Geometry: final body of the model. Coordinates: model frame, mm. A direction names the side the tool comes from. Coordinates: 2 decimals unless noted, no trailing zeros. Loops run counter-clockwise (first coordinate to the right, second up) from the corner with the lowest first, then second, coordinate; pieces in that order, holes last. Notation, with made-up numbers: (-28.5, 81.5) - (17.5, 81.5) arc R27 cw to (17.5, 110.5) - close; hole circle Ø7 at (-34.75, 46.25). An arc over 180 degrees is marked (long way). Return JSON: item names as keys, results as strings.
from build123d import *

# Parameters (mm, degrees)
EXTRUDE_THIN1_DEPTH    = 16.002
CUT_EXTRUDE1_START     = -15.748
CUT_EXTRUDE1_OUTLINE_R = 1.3
CUT_EXTRUDE1_DEPTH     = 15.748
BOSS_EXTRUDE2_DEPTH    = 1.68
BOSS_EXTRUDE3_START    = 1.68
BOSS_EXTRUDE3_DEPTH    = 1.68
CUT_EXTRUDE2_START     = -2.384
CUT_EXTRUDE2_DEPTH     = 2.384
CUT_EXTRUDE3_DEPTH     = 2.384
CHAMFER1_SIZE          = 1.7
CHAMFER2_SIZE          = 2.38


# Read off the part's stored shape, not the designer's step: Cut-Extrude1
with BuildPart() as part:
    # Sketch1 → Extrude-Thin1 (new body)
    with BuildSketch(Plane.XY):
        with BuildLine():
            Line((-42.06875, -12.7), (-35.433, -12.7))
            ThreePointArc((-35.433, -12.7), (-33.636948776, -11.956051224), (-32.893, -10.16))
            Line((-32.893, -10.16), (-32.893, -2.54))
            ThreePointArc((-32.893, -2.54), (-32.149051224, -0.743948776), (-30.353, 0))
            Line((-30.353, 0), (30.353, 0))
            ThreePointArc((30.353, 0), (32.149051224, -0.743948776), (32.893, -2.54))
            Line((32.893, -2.54), (32.893, -10.16))
            ThreePointArc((32.893, -10.16), (33.636948776, -11.956051224), (35.433, -12.7))
            Line((35.433, -12.7), (42.06875, -12.7))
            Line((42.06875, -12.7), (42.06875, -15.748))
            Line((42.06875, -15.748), (35.433, -15.748))
            ThreePointArc((35.433, -15.748), (31.481687307, -14.111312693), (29.845, -10.16))
            Line((29.845, -10.16), (29.845, -3.048))
            Line((29.845, -3.048), (-29.845, -3.048))
            Line((-29.845, -3.048), (-29.845, -10.16))
            ThreePointArc((-29.845, -10.16), (-31.481687307, -14.111312693), (-35.433, -15.748))
            Line((-35.433, -15.748), (-42.06875, -15.748))
            Line((-42.06875, -15.748), (-42.06875, -12.7))
        make_face()
    extrude(amount=-EXTRUDE_THIN1_DEPTH)

    # Cut-Extrude1 outline → Cut-Extrude1 (cut)
    with BuildSketch(Plane(origin=(0, 0, 0), x_dir=(1, 0, 0), z_dir=(0, 1, 0)).offset(CUT_EXTRUDE1_START)):
        with BuildLine():
            Line((35.433, 13.462), (-35.433, 13.462))
            ThreePointArc((-35.433, 13.462), (-37.133, 11.762), (-35.433, 10.062))
            Line((-35.433, 10.062), (-32.893, 10.062))
            Line((-32.893, 10.062), (-32.893, 8.382))
            Line((-32.893, 8.382), (-1.27, 8.382))
            Line((-1.27, 8.382), (-1.27, 12.446))
            Line((-1.27, 12.446), (32.893, 12.446))
            Line((32.893, 12.446), (32.893, 10.062))
            Line((32.893, 10.062), (35.433, 10.062))
            ThreePointArc((35.433, 10.062), (37.133, 11.762), (35.433, 13.462))
        make_face()
        with BuildLine():
            Line((32.893, 5.94), (32.893, 7.62))
            Line((32.893, 7.62), (1.27, 7.62))
            Line((1.27, 7.62), (1.27, 3.556))
            Line((1.27, 3.556), (-32.893, 3.556))
            Line((-32.893, 3.556), (-32.893, 5.94))
            Line((-32.893, 5.94), (-35.433, 5.94))
            ThreePointArc((-35.433, 5.94), (-37.133, 4.24), (-35.433, 2.54))
            Line((-35.433, 2.54), (35.433, 2.54))
            ThreePointArc((35.433, 2.54), (37.133, 4.24), (35.433, 5.94))
            Line((35.433, 5.94), (32.893, 5.94))
        make_face()
        with BuildLine():
            Line((42.06875, 16.002), (35.433, 16.002))
            ThreePointArc((35.433, 16.002), (40.193949205, 13.198335352), (42.06875, 8.001))
            Line((42.06875, 8.001), (42.06875, 16.002))
        make_face()
        with BuildLine():
            Line((42.06875, 0), (42.06875, 8.001))
            ThreePointArc((42.06875, 8.001), (40.193949205, 2.803664648), (35.433, 0))
            Line((35.433, 0), (42.06875, 0))
        make_face()
        with BuildLine():
            ThreePointArc((-42.06875, 8.001), (-40.193949205, 13.198335352), (-35.433, 16.002))
            Line((-35.433, 16.002), (-42.06875, 16.002))
            Line((-42.06875, 16.002), (-42.06875, 8.001))
        make_face()
        with BuildLine():
            ThreePointArc((-35.433, 0), (-40.193949205, 2.803664648), (-42.06875, 8.001))
            Line((-42.06875, 8.001), (-42.06875, 0))
            Line((-42.06875, 0), (-35.433, 0))
        make_face()
        with Locations((38.750875, 8.001)):
            Circle(CUT_EXTRUDE1_OUTLINE_R)
        with Locations((-38.750875, 8.001)):
            Circle(CUT_EXTRUDE1_OUTLINE_R)
    extrude(amount=CUT_EXTRUDE1_DEPTH, mode=Mode.SUBTRACT)

    # Sketch6 → Boss-Extrude2 (add)
    with BuildSketch(Plane(origin=(0, 0, -8.382), x_dir=(-1, 0, 0), z_dir=(0, 0, -1))):
        with BuildLine():
            Line((32.893, -10.16), (32.893, -6.604))
            Line((32.893, -6.604), (29.845, -6.604))
            Line((29.845, -6.604), (29.845, -10.16))
            ThreePointArc((29.845, -10.16), (30.667537588, -13.078237824), (32.893, -15.137363157))
            Line((32.893, -15.137363157), (32.893, -10.16))
        make_face()
    extrude(amount=BOSS_EXTRUDE2_DEPTH)

    # Sketch7 → Boss-Extrude3 (add)
    with BuildSketch(Plane.XY.offset(-7.62).offset(BOSS_EXTRUDE3_START)):
        with BuildLine():
            Line((32.893, -10.16), (32.893, -6.6))
            Line((32.893, -6.6), (29.845, -6.604))
            Line((29.845, -6.604), (29.845, -10.16))
            ThreePointArc((29.845, -10.16), (30.667537588, -13.078237824), (32.893, -15.137363157))
            Line((32.893, -15.137363157), (32.893, -10.16))
        make_face()
    extrude(amount=-BOSS_EXTRUDE3_DEPTH)

    # Sketch8 → Cut-Extrude2 (cut)
    with BuildSketch(Plane(origin=(0, 0, -12.446), x_dir=(-1, 0, 0), z_dir=(0, 0, -1)).offset(CUT_EXTRUDE2_START)):
        with BuildLine():
            Line((-32.893, -15.137363157), (-32.893, -6.6))
            Line((-32.893, -6.6), (-29.845, -6.604))
            Line((-29.845, -6.604), (-29.845, -10.16))
            ThreePointArc((-29.845, -10.16), (-30.667537588, -13.078237824), (-32.893, -15.137363157))
        make_face()
    extrude(amount=CUT_EXTRUDE2_DEPTH, mode=Mode.SUBTRACT)

    # Sketch9 → Cut-Extrude3 (cut)
    with BuildSketch(Plane.XY.offset(-3.556)):
        with BuildLine():
            Line((-32.893, -15.137363157), (-32.893, -6.604))
            Line((-32.893, -6.604), (-29.845, -6.604))
            Line((-29.845, -6.604), (-29.845, -10.16))
            ThreePointArc((-29.845, -10.16), (-30.667537588, -13.078237824), (-32.893, -15.137363157))
        make_face()
    extrude(amount=-CUT_EXTRUDE3_DEPTH, mode=Mode.SUBTRACT)

    # Chamfer1
    # the kernel refuses this chamfer: 1.7 mm, written as the material it adds along each edge
    # the kernel refuses this chamfer: 1.7 mm, written as the material it takes off along each edge
    with BuildSketch(Plane(origin=(-37.26486108, -6.604, -10.062), x_dir=(0, -0.9996219169112968, -0.02749587661058687), z_dir=(1, 0, 0))) as chamfer1_2_piece_1_section:
        Polygon((CHAMFER1_SIZE * 0.999621916911, -CHAMFER1_SIZE * 0.0274958766106), (-CHAMFER1_SIZE * 0.0274958766106, -CHAMFER1_SIZE * 0.999621916911), (0, 0), align=None)
    chamfer1_2_piece_1 = extrude(amount=11.791722159, mode=Mode.PRIVATE)
    chamfer1_2_piece_1 = split(chamfer1_2_piece_1, bisect_by=Plane(origin=(-31.369, -7.170744186, -8.382), z_dir=(0, 0, -1)), keep=Keep.TOP, mode=Mode.PRIVATE)
    add(chamfer1_2_piece_1, mode=Mode.SUBTRACT)
    with BuildSketch(Plane(origin=(37.264857315, -6.594262654, -5.94), x_dir=(0.00131183865632537, -0.9996210561251475, 0.02749587661058631), z_dir=(-0.999999138888279, -0.0013123348279305267, 0))) as chamfer1_2_piece_2_section:
        Polygon((CHAMFER1_SIZE * 0.999621916911, -CHAMFER1_SIZE * 0.0274958766106), (-CHAMFER1_SIZE * 0.0274958766106, -CHAMFER1_SIZE * 0.999621916911), (0, 0), align=None)
    chamfer1_2_piece_2 = extrude(amount=11.791724784, mode=Mode.PRIVATE)
    chamfer1_2_piece_2 = split(chamfer1_2_piece_2, bisect_by=Plane(origin=(31.369, -7.168744674, -7.62), z_dir=(0, 0, 1)), keep=Keep.TOP, mode=Mode.PRIVATE)
    add(chamfer1_2_piece_2, mode=Mode.SUBTRACT)

    # Chamfer2
    chamfer2_edges = [part.edges().sort_by_distance(p)[0] for p in [
        (31.369, -6.602, -10.062),
        (-31.369, -6.604, -5.94),
    ]]
    chamfer(chamfer2_edges, length=CHAMFER2_SIZE)


solid = part.part
Item 1: Section query B-B, the plane y = -13.5. Return loops of the section in (x, z), and give its area (3 significant figures).
Worked out:
{"outline": "(-35.43, -16) - (-30.95, -16) - (-30.95, -13.46) - (-35.43, -13.46) arc R1.7 cw to (-35.43, -10.06) - (-30.95, -10.06) - (-30.95, -5.94) - (-35.43, -5.94) arc R1.7 cw to (-35.43, -2.54) - (-30.95, -2.54) - (-30.95, 0) - (-35.43, 0) arc R8.14 ccw to start; (30.95, -16) - (35.43, -16) arc R8.14 ccw to (35.43, 0) - (30.95, 0) - (30.95, -2.54) - (35.43, -2.54) arc R1.7 cw to (35.43, -5.94) - (30.95, -5.94) - (30.95, -10.06) - (35.43, -10.06) arc R1.7 cw to (35.43, -13.46) - (30.95, -13.46) - close; hole circle Ø2.6 at (-38.75, -8); hole circle Ø2.6 at (38.75, -8)", "area": "213 mm^2"}
Item 2: Section query A-A, the plane y = -5.25. Return loops of the section in (x, z) (3 decimals).
Worked out:
{"outline": "(-32.893, -16.002) - (-29.845, -16.002) - (-29.845, -13.462) - (-32.893, -13.462) - close; (-32.893, -8.382) - (-29.845, -8.382) - (-29.845, -3.556) - (-32.893, -3.556) - close; (-32.893, -2.54) - (-29.845, -2.54) - (-29.845, 0) - (-32.893, 0) - close; (29.845, -16.002) - (32.893, -16.002) - (32.893, -13.462) - (29.845, -13.462) - close; (29.845, -12.446) - (32.893, -12.446) - (32.893, -7.62) - (29.845, -7.62) - close; (29.845, -2.54) - (32.893, -2.54) - (32.893, 0) - (29.845, 0) - close"}
Item 3: Ray query, probe 1 along Z at (x, y) = (31.5, -2.5); probe 2 along Y at (x, z) = (13, -11); probe 3 along X at (y, z) = (-2.25, -12). Return the intervals inside material, ascending. Write a range as from..to.
Worked out:
{"probe 1": "-16..-13.46, -12.45..-7.62, -2.54..0", "probe 2": "-3.05..0", "probe 3": "-1.27..32.88"}
Item 4: Reachability of faces 1 (the face through (1.27, -2, -6)), 2 (the face through (32.893, -6, -9)), 3 (the face through (-31.39, -7.476, -9.234)), 4 (the face through (-33, -12, -10.062)), 5 (the face through (29.845, -7, -15)) from +Z, -Z, +X, -X, +Y, -Y: full face, straight path, thin tool, end or side. Return the list, or none.
Worked out:
{"face 1": "+X, +Y, -Y", "face 2": "+Z, -Z, +X, +Y", "face 3": "-X, +Y", "face 4": "+Y, -Y", "face 5": "+Z, -Z, -Y"}
Item 5: Section query C-C, the plane x = -7.5. Return loops of the section in (y, z), and give its area (3 significant figures).
Worked out:
{"outline": "(-3.05, -16) - (0, -16) - (0, -13.46) - (-3.05, -13.46) - close; (-3.05, -8.38) - (0, -8.38) - (0, -3.56) - (-3.05, -3.56) - close; (-3.05, -2.54) - (0, -2.54) - (0, 0) - (-3.05, 0) - close", "area": "30.2 mm^2"}
Item 6: Section query D-D, the plane y = -1.5. Return loops of the section in (x, z).
Worked out:
{"outline": "(-32.67, -16) - (32.67, -16) - (32.67, -13.46) - (-32.67, -13.46) - close; (-32.67, -8.38) - (-1.27, -8.38) - (-1.27, -12.45) - (32.67, -12.45) - (32.67, -7.62) - (1.27, -7.62) - (1.27, -3.56) - (-32.67, -3.56) - close; (-32.67, -2.54) - (32.67, -2.54) - (32.67, 0) - (-32.67, 0) - close"}
Item 7: First-contact query: pin 1 Ø8 at (y, z) = (-4, -9) entering from +X; pin 2 Ø6 at (x, z) = (-1.5, -8) entering from -Y; pin 3 Ø0.8 at (y, z) = (-8, -1) entering from -X. Flat tips, straight axial feed; report the tip coordinate or a pass-through.
Worked out:
{"pin 1": "x = 32.89", "pin 2": "y = -3.05", "pin 3": "x = -32.89"}
Item 8: Mould query, pull axis X, two halves, no side actions, for faces 6 (the face through (37, -15.748, -8)), 7 (the face through (33.62, -11.94, -14.71)), 8 (the face through (-29.845, -7, -1)). Classes: +X half, -X half, draft (parallel to the pull), parting line (faces both ways), or undercut.
Worked out:
{"face 6": "draft", "face 7": "+X half", "face 8": "undercut"}
